For this review, take the finished solid that the model builds, in its own axes (mm). Face numbers are marked on the shaded views. A direction names the side the tool comes from. Give positions to 0.01 mm unless a question says otherwise; leave off trailing zeros. Write each loop counter-clockwise with the first axis right and the second up, starting at its lowest first coordinate (ties: lowest second). Pieces come first, ordered by that corner, then holes.
Q1. Insertion check: P1, Ø12, axis at y = -10.5, z = -2.5, coming from the -X side; P2, Ø1, axis at x = -1, z = 2.5, coming from the -Y side; P3, Ø2, axis at x = -1, z = -7, coming from the -Y side; P4, Ø4, axis at x = 1.5, y = -14, coming from the -Z side. Each pin has a flat end and moves straight along its axis. Give the tip position at first contact, or say it passes through.
Q2. We need section A-A (x = 0). Write out the cut boundary in (y, z).
Q3. Mouldability with a two-part tool opening along Y and no side actions: class the marked faces 1, 2 and 3 as released by +Y, released by -Y, zero draft, split by the parting line, or undercut.
Q4. We need section D-D (y = 2.5). Write out the cut boundary in (x, z).
Q5. For line 1 (X direction, y = 4, z = -10); line 2 (Y direction, x = 0, z = 5); line 3 (Y direction, x = -2.75, z = -12.5), list the stretches that pass through material, from the lowest coordinate up.
Q6. We need section C-C (z = -11). Write out the cut boundary in (x, y).
Q7. We need section B-B (y = -15.75). Write out the cut boundary in (x, z).
Q8. Machinability: for the marked faces 4 and 5, which of the approach directions +Z, -Z, +X, -X, +Y, -Y give a long, thin tool a straight path to every point of the face, cutting with its end or side? Answer none if there is none.
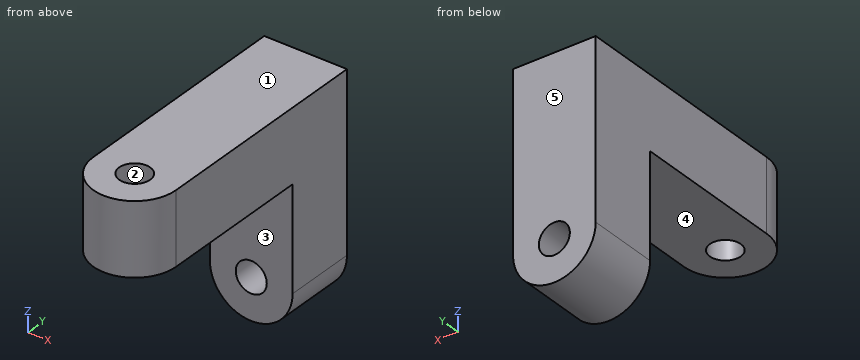
```python
from build123d import *

# Parameters (mm, degrees)
SKETCH2_R           = 1.5
BOSS_EXTRUDE1_DEPTH = 7
SKETCH3_R           = 1.5
BOSS_EXTRUDE2_DEPTH = 7


with BuildPart() as part:
    # Sketch2 → Boss-Extrude1 (new body)
    with BuildSketch(Plane.XY):
        with BuildLine():
            Line((-4, -15), (-4, 0))
            Line((-4, 0), (4, 0))
            Line((4, 0), (4, -15))
            ThreePointArc((4, -15), (0, -19), (-4, -15))
        make_face()
        with Locations((0, -15)):
            Circle(SKETCH2_R, mode=Mode.SUBTRACT)
    extrude(amount=BOSS_EXTRUDE1_DEPTH)

    # Sketch3 → Boss-Extrude2 (add)
    with BuildSketch(Plane(origin=(0, 0, 0), x_dir=(1, 0, 0), z_dir=(0, 1, 0))):
        with BuildLine():
            Line((-4, 10), (-4, -7))
            Line((-4, -7), (4, -7))
            Line((4, -7), (4, 10))
            ThreePointArc((4, 10), (0, 14), (-4, 10))
        make_face()
        with Locations((0, 10)):
            Circle(SKETCH3_R, mode=Mode.SUBTRACT)
    extrude(amount=BOSS_EXTRUDE2_DEPTH)


solid = part.part
```
Computed:
1. P1: stops at x = -4
1. P2: stops at y = -18.97
1. P3: stops at y = 0
1. P4: stops at z = 0
2. outline: (-19, 0) - (-16.5, 0) - (-16.5, 7) - (-19, 7) - close; (-13.5, 0) - (0, 0) - (0, -8.5) - (7, -8.5) - (7, 7) - (-13.5, 7) - close; (0, -14) - (7, -14) - (7, -11.5) - (0, -11.5) - close
3. face 1: zero draft
3. face 2: undercut
3. face 3: released by -Y
4. outline: (-4, -10) arc R4 ccw to (4, -10) - (4, 7) - (-4, 7) - close; hole circle Ø3 at (0, -10)
5. line 1: x = -4 to -1.5, 1.5 to 4
5. line 2: y = -19 to -16.5, -13.5 to 7
5. line 3: y = 0 to 7
6. outline: (-3.87, 0) - (-1.12, 0) - (-1.12, 7) - (-3.87, 7) - close; (1.12, 0) - (3.87, 0) - (3.87, 7) - (1.12, 7) - close
7. outline: (-3.93, 0) - (-1.3, 0) - (-1.3, 7) - (-3.93, 7) - close; (1.3, 0) - (3.93, 0) - (3.93, 7) - (1.3, 7) - close
8. face 4: -Z, +X, -X, -Y
8. face 5: +Z, -Z, +X, -X, +Y
